Check sheet for the modelled part. Datum: model origin and axes. Units: mm. A direction names the side the tool comes from. Round coordinates to 2 decimals unless told otherwise and drop trailing zeros. Order: outer loops, then holes, each group sorted by start corner. A loop starts at its lowest first (then second) coordinate and runs counter-clockwise, first axis right, second up.
Q1. Set-up check for faces 1 (the cylindrical face through (14.86, -29.97, 1.32)), 2 (the cylindrical face through (43, 29, 0)), 3 (the flat face through (247, 25.7, -4)): record each of +Z, -Z, +X, -X, +Y, -Y from which the full face is reachable in a straight line by a thin tool's end or side.
Q2. Cross-section at A-A on x = 179. Record the cut outline in (y, z).
Q3. Depth check by flat-ended pin: P1, Ø1.5, axis at x = 255.5, y = 27, coming from the +Z side; P2, Ø5, axis at x = 175.5, y = 11, coming from the +Z side; P3, Ø1.5, axis at x = 160, y = -21, coming from the +Z side. Enter the tip coordinate at first touch or a pass-through.
Q4. Scan lines: probe 1 along X at (y, z) = (22, 0); probe 2 along Y at (x, z) = (15, 1); probe 3 along Z at (x, y) = (247, 23). Record each from-to range of solid material in increasing order.
from build123d import *

# Parameters (mm, degrees)
CHAMFER1_SIZE                  = 1
CUT_EXTRUDE1_REACH             = 8.8
F_5_0MM_DOWEL_HOLE1_D          = 4.2
F_5_0MM_DOWEL_HOLE1_DEPTH      = 5
F_5_0MM_DOWEL_HOLE1_TIP        = 1.2618073
CUT_EXTRUDE2_REACH             = 34.5
CUT_EXTRUDE2_DIRECTION_2_REACH = 34.5


with BuildPart() as part:
    # Sketch1 → Revolve1 (revolve)
    with BuildSketch(Plane.XY):
        with BuildLine():
            Line((0, 0), (272, 0))
            Line((272, 0), (272, 30))
            Line((272, 30), (129, 30))
            Line((129, 30), (127.954891423, 29.719964001))
            ThreePointArc((127.954891423, 29.719964001), (127.182150762, 29.927019237), (126.975095526, 30.699759898))
            Line((126.975095526, 30.699759898), (127, 30.792704662))
            Line((127, 30.792704662), (127, 32.5))
            Line((127, 32.5), (27, 32.5))
            Line((27, 32.5), (27, 30.792704662))
            Line((27, 30.792704662), (27.024904474, 30.699759898))
            ThreePointArc((27.024904474, 30.699759898), (26.817849238, 29.927019237), (26.045108577, 29.719964001))
            Line((26.045108577, 29.719964001), (25, 30))
            Line((25, 30), (5, 30))
            Line((5, 30), (5, 28.5))
            Line((5, 28.5), (2.85, 28.5))
            Line((2.85, 28.5), (2.85, 30))
            Line((2.85, 30), (0, 30))
            Line((0, 30), (0, 0))
        make_face()
    revolve(axis=Axis((0, 0, 0), (1, 0, 0)))

    # Chamfer1
    chamfer1_edges = [part.edges().sort_by_distance(p)[0] for p in [
        (272, -30, 0),
        (127, -32.5, 0),
        (27, -32.5, 0),
        (0, -30, 0),
    ]]
    chamfer(chamfer1_edges, length=CHAMFER1_SIZE)

    # Sketch2 → Cut-Extrude1 (cut, up to next)
    with BuildSketch(Plane(origin=(0, 25.7, 0), x_dir=(1, 0, 0), z_dir=(0, 1, 0)), mode=Mode.PRIVATE) as cut_extrude1_sk1:
        Polygon((272, 9), (222, 9), (222, -9), (272, -9), (272, 0), align=None)
    cut_extrude1_tool1 = extrude(cut_extrude1_sk1.sketch, amount=CUT_EXTRUDE1_REACH, mode=Mode.PRIVATE) & part.part
    add(cut_extrude1_tool1.solids().sort_by_distance((247, 25.7, 0))[0], mode=Mode.SUBTRACT)
    # Sketch2 → Cut-Extrude1 (cut, up to next)
    with BuildSketch(Plane(origin=(0, 25.7, 0), x_dir=(1, 0, 0), z_dir=(0, 1, 0)), mode=Mode.PRIVATE) as cut_extrude1_sk2:
        with BuildLine():
            Line((52, 9), (102, 9))
            ThreePointArc((102, 9), (111, 0), (102, -9))
            Line((102, -9), (52, -9))
            ThreePointArc((52, -9), (43, 0), (52, 9))
        make_face()
    cut_extrude1_tool2 = extrude(cut_extrude1_sk2.sketch, amount=CUT_EXTRUDE1_REACH, mode=Mode.PRIVATE) & part.part
    add(cut_extrude1_tool2.solids().sort_by_distance((77, 25.7, 0))[0], mode=Mode.SUBTRACT)

    # Ø5.0mm Dowel Hole1
    with Locations(Plane(origin=(247, 25.7, 0), x_dir=(0, 0, 1), z_dir=(0, 1, 0))):
        with Locations((0, 0)):
            Hole(F_5_0MM_DOWEL_HOLE1_D / 2, depth=F_5_0MM_DOWEL_HOLE1_DEPTH)
            with Locations((0, 0, -(F_5_0MM_DOWEL_HOLE1_DEPTH + F_5_0MM_DOWEL_HOLE1_TIP / 2))):  # 118° drill point
                Cone(0, F_5_0MM_DOWEL_HOLE1_D / 2, F_5_0MM_DOWEL_HOLE1_TIP, mode=Mode.SUBTRACT)

    # Cut-Extrude2: up to this face of the body (flat: up to its plane)
    cut_extrude2_end = Plane(part.part.faces().sort_by_distance((246.910970255, 27.155084714, -9))[0])
    # Sketch5 → Cut-Extrude2 (cut, up to the picked face)
    with BuildSketch(Plane.XY, mode=Mode.PRIVATE) as cut_extrude2_sk1:
        with BuildLine():
            Line((222, 30), (222, 25.7))
            ThreePointArc((222, 25.7), (216.557344398, 26.820568368), (212, 30))
            Line((212, 30), (222, 30))
        make_face()
    cut_extrude2_tool1 = split(extrude(cut_extrude2_sk1.sketch, amount=-CUT_EXTRUDE2_REACH, mode=Mode.PRIVATE), bisect_by=cut_extrude2_end, keep=Keep.BOTH, mode=Mode.PRIVATE)
    add(cut_extrude2_tool1.solids().sort_by_distance((218.157433, 28.254696, 0))[0], mode=Mode.SUBTRACT)

    # Cut-Extrude2 direction 2: up to this face of the body (flat: up to its plane)
    cut_extrude2_direction_2_end = Plane(part.part.faces().sort_by_distance((246.910970255, 27.155084714, 9))[0])
    # Sketch5 → Cut-Extrude2 direction 2 (cut, up to the picked face)
    with BuildSketch(Plane.XY, mode=Mode.PRIVATE) as cut_extrude2_direction_2_sk1:
        with BuildLine():
            Line((222, 30), (222, 25.7))
            ThreePointArc((222, 25.7), (216.557344398, 26.820568368), (212, 30))
            Line((212, 30), (222, 30))
        make_face()
    cut_extrude2_direction_2_tool1 = split(extrude(cut_extrude2_direction_2_sk1.sketch, amount=CUT_EXTRUDE2_DIRECTION_2_REACH, mode=Mode.PRIVATE), bisect_by=cut_extrude2_direction_2_end, keep=Keep.BOTH, mode=Mode.PRIVATE)
    add(cut_extrude2_direction_2_tool1.solids().sort_by_distance((218.157433, 28.254696, 0))[0], mode=Mode.SUBTRACT)


solid = part.part
Results found:
1. face 1: -X
1. face 2: +Y
1. face 3: +X, +Y
2. outline: circle Ø60 at (0, 0)
3. P1: stops at z = 14.52
3. P2: stops at z = 28.77
3. P3: stops at z = 22.13
4. probe 1: x = 0 to 244.9, 249.1 to 272
4. probe 2: y = -29.98 to 29.98
4. probe 3: z = -19.26 to -2.1, 2.1 to 19.26
